Study the drawing (mm; zero at the part's minimum x, y, z) and answer. Give positions to 0.01 mm unless a question says otherwise; leave off trailing zeros. Loops run counter-clockwise (first coordinate to the right, second up) from the corner with the lowest first, then second, coordinate; pieces in that order, holes last. Notation, with made-up numbers: (19, -34) - (72, -34) arc R25 ccw to (72, 4) - close; hole circle Ø10 at (40, -37). An arc over 180 degrees is marked (long way). Use one line per item in the form item = value. Start each with the question number.
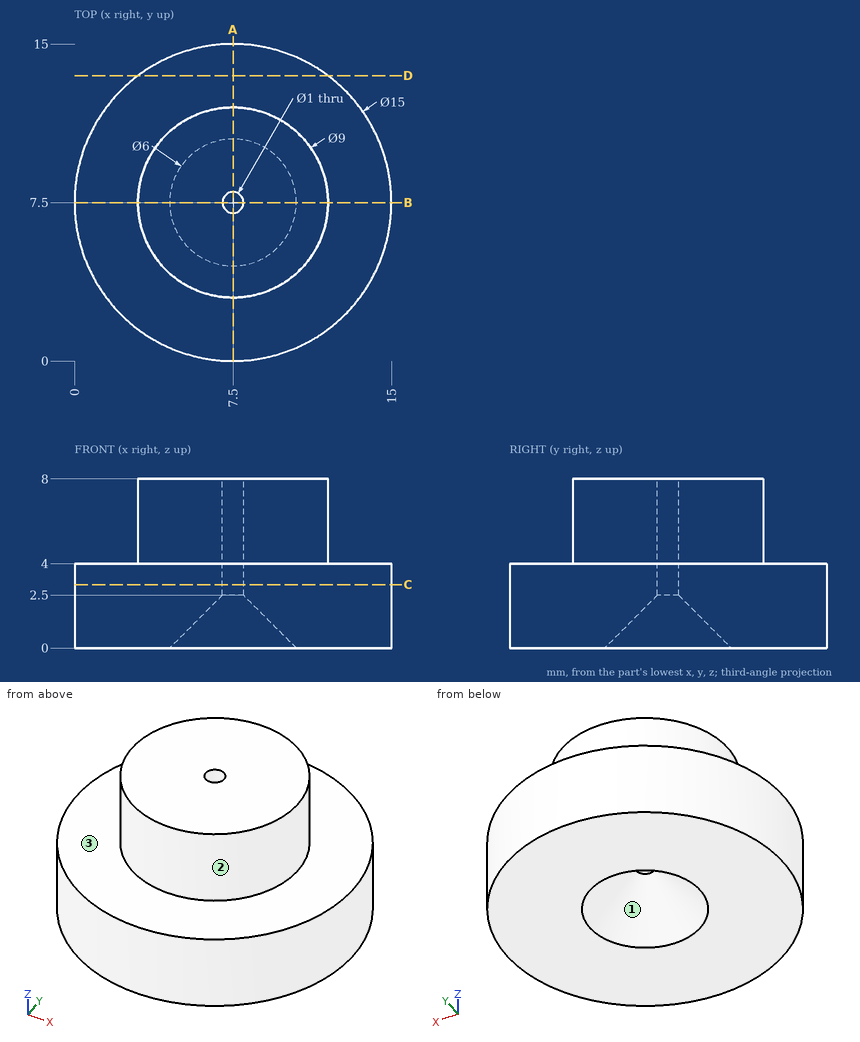
1) A cutting plane is placed at D-D (y = 13.5). Give the vertices of the cut face in (x, z), plus the area to 3 significant figures.
2) Find the intervals of material crossed by probe 1 along Y at (x, z) = (7.5, 5.15); probe 2 along Z at (x, y) = (10.25, 12.5), in increasing order.
3) Determine the mould class of the marked faces 1, 2 and 3 for opening direction Y: released by +Y, released by -Y, zero draft, split by the parting line, or undercut.
4) A cutting plane is placed at A-A (x = 7.5). Give the vertices of the cut face in (y, z).
5) A cutting plane is placed at C-C (z = 3). Give the vertices of the cut face in (x, y).
Answer sheet:
q1.outline = (3, 0) - (12, 0) - (12, 4) - (3, 4) - close
q1.area = 36.0 mm²
q2.probe_1 = 3 to 7, 8 to 12
q2.probe_2 = 0 to 4
q3.face_1 = undercut
q3.face_2 = split by the parting line
q3.face_3 = zero draft
q4.outline = (0, 0) - (4.5, 0) - (7, 2.5) - (7, 8) - (3, 8) - (3, 4) - (0, 4) - close; (8, 2.5) - (10.5, 0) - (15, 0) - (15, 4) - (12, 4) - (12, 8) - (8, 8) - close
q5.outline = circle Ø15 at (7.5, 7.5); hole circle Ø1 at (7.5, 7.5)
